Build history of the part. All positions in model axes, mm. A direction names the side the tool comes from. Coordinates: 2 decimals unless noted, no trailing zeros. One line per item, written item: value.
```python
from build123d import *

# Parameters (mm, degrees)
F0_W     = 6.35
F0_H     = 6.35
F0_R     = 1.8415
F1_DEPTH = 78.1375882
F2_DEPTH = 6.35
F4_START = 1.0583333333
F3_W     = 6.35
F3_H     = 7.14375
F3_R     = 0.635
F4_DEPTH = 2.1166666667


with BuildPart() as f1:
    # F0 (on Top) → F1 (new body)
    with BuildSketch(Plane.XY):
        Rectangle(F0_W, F0_H)
        Circle(F0_R, mode=Mode.SUBTRACT)
        Circle(F0_R)
    extrude(amount=F1_DEPTH)

    # F0 (on Top) → F2 (cut)
    with BuildSketch(Plane.XY):
        Circle(F0_R)
    extrude(amount=F2_DEPTH, mode=Mode.SUBTRACT)

    # F3 (on Right) → F4 (join)
    with BuildSketch(Plane.YZ.offset(F4_START)):
        with Locations((0, 81.7094632)):
            Rectangle(F3_W, F3_H)
        with Locations((0, 81.7094632)):
            Circle(F3_R, mode=Mode.SUBTRACT)
    extrude(amount=F4_DEPTH)


solid = f1.part
```
Item 1: Pull direction Y, two halves, no side cores. Call faces 4 (the face through (1.4, 1.5, 0)), 5 (the face through (0, 0, 6.35)), 6 (the face through (0, -3.175, 42)): released by +Y, released by -Y, zero draft, split by the parting line, or undercut.
Check result:
face 4: zero draft
face 5: undercut
face 6: released by -Y
Item 2: Tool access for faces 1 (the face through (0.85, -1.634, 3.131)), 2 (the face through (2, 0, 85.281)), 3 (the face through (-1, 0, 78.138)): list every direction of +Z, -Z, +X, -X, +Y, -Y with a clear straight run to the whole face (end or side of a thin tool).
Check result:
face 1: -Z
face 2: +Z, +X, -X, +Y, -Y
face 3: +Z, -X, +Y, -Y
Item 3: Drop flat-ended pins along their axis: P1, Ø1, axis at x = -2, y = -0.5, coming from the +Z side; P2, Ø3, axis at y = -1.5, z = 81.5, coming from the -X side; P3, Ø2, axis at x = 0, y = 0, coming from the -Z side. Give the stop position or say it passes through.
Check result:
P1: stops at z = 78.14
P2: stops at x = 1.06
P3: stops at z = 6.35
Item 4: Probe probe 1 along Z at (x, y) = (2.05, 0); probe 2 along Y at (x, z) = (0, 3) (1 decimal); probe 3 along Z at (x, y) = (-0.75, -0.75). List the from-to ranges inside material, lowest first. Write a range as from..to.
Check result:
probe 1: z = 0..81.07, 82.34..85.28
probe 2: y = -3.2..-1.8, 1.8..3.2
probe 3: z = 6.35..78.14
